```python
from build123d import *

# Parameters (mm, degrees)
ESBO_O1_R                = 2.5
RESSALTO_EXTRUS_O1_DEPTH = 6
ESBO_O2_W                = 13.5
ESBO_O2_H                = 13.5
RESSALTO_EXTRUS_O2_DEPTH = 6
FILETE1_R                = 8
ESBO_O3_R                = 1.5
CORTE_EXTRUS_O1_DEPTH    = 6


with BuildPart() as part:
    # Esboço1 → Ressalto-extrusão1 (new body)
    with BuildSketch(Plane.XY):
        with BuildLine():
            Line((-20, 33.5), (20, 33.5))
            ThreePointArc((20, 33.5), (29.545941546, 29.545941546), (33.5, 20))
            Line((33.5, 20), (33.5, -20))
            ThreePointArc((33.5, -20), (29.545941546, -29.545941546), (20, -33.5))
            Line((20, -33.5), (-20, -33.5))
            ThreePointArc((-20, -33.5), (-29.545941546, -29.545941546), (-33.5, -20))
            Line((-33.5, -20), (-33.5, 20))
            ThreePointArc((-33.5, 20), (-29.545941546, 29.545941546), (-20, 33.5))
        make_face()
        with Locations((-20, 20)):
            Circle(ESBO_O1_R, mode=Mode.SUBTRACT)
        with Locations((20, 20)):
            Circle(ESBO_O1_R, mode=Mode.SUBTRACT)
        with Locations((0, -20)):
            Circle(ESBO_O1_R, mode=Mode.SUBTRACT)
    extrude(amount=RESSALTO_EXTRUS_O1_DEPTH)

    # Esboço2 → Ressalto-extrusão2 (add)
    with BuildSketch(Plane(origin=(0, 0, 0), x_dir=(-1, 0, 0), z_dir=(0, 0, -1))):
        with Locations((-26.75, -26.75)):
            Rectangle(ESBO_O2_W, ESBO_O2_H)
        with Locations((26.75, -26.75)):
            Rectangle(ESBO_O2_W, ESBO_O2_H)
    extrude(amount=-RESSALTO_EXTRUS_O2_DEPTH)

    # Filete1
    filete1_edges = [part.edges().sort_by_distance(p)[0] for p in [
        (33.5, -33.5, 3),
        (-33.5, -33.5, 3),
    ]]
    fillet(filete1_edges, radius=FILETE1_R)

    # Esboço3 → Corte-extrusão1 (cut)
    with BuildSketch(Plane(origin=(0, 0, 0), x_dir=(-1, 0, 0), z_dir=(0, 0, -1))):
        with Locations((0, 20)):
            Circle(ESBO_O3_R)
        with Locations((20, -20)):
            Circle(ESBO_O3_R)
        with Locations((-20, -20)):
            Circle(ESBO_O3_R)
    extrude(amount=-CORTE_EXTRUS_O1_DEPTH, mode=Mode.SUBTRACT)


solid = part.part
```
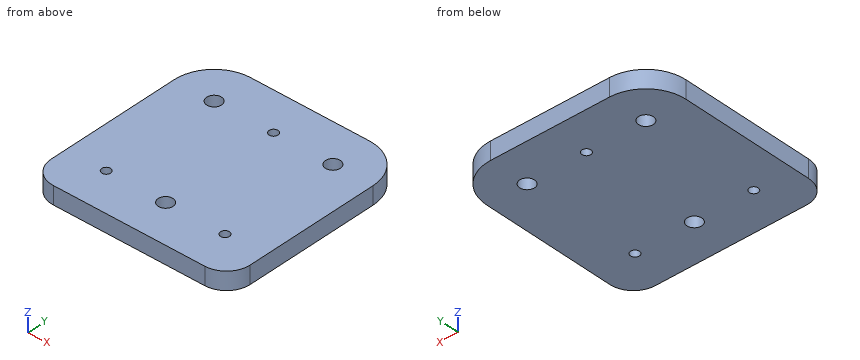
Verification items for the finished model (mm, model axes). Give positions to 0.01 mm unless a question says otherwise; leave off trailing zeros. Order: outer loops, then holes, each group sorted by start corner. A loop starts at its lowest first (then second) coordinate and runs counter-clockwise, first axis right, second up. Notation, with made-up numbers: (67.25, 59.25) -> (111.25, 59.25) arc R18 ccw to (111.25, 64.25) -> close; hole circle Ø3 at (54, 43). An arc over 180 degrees is marked (long way). One line per item, written item: value.
(1) Gauge pin test, flat end, axial feed: pin 1 (1.8 mm diameter, centred on x = 0, y = 20, fed in from -Z). Record the tip position at first contact, or that the pin passes through.
Final values:
pin 1: through
(2) Scan lines: line 1 along Y through (x, z) = (0, 2.85); line 2 along Y through (x, z) = (-20, 4.5); line 3 along X through (y, z) = (-18, 2). Record each from-to range of solid material in increasing order. Write a range as [from, to].
Final values:
line 1: [-33.5, -22.5], [-17.5, 18.5], [21.5, 33.5]
line 2: [-33.5, -21.5], [-18.5, 17.5], [22.5, 33.5]
line 3: [-33.5, -1.5], [1.5, 33.5]
(3) Sectioned sample at B-B on y = -20. Record the cut outline in (x, z).
Final values:
outline: (-33.5, 0) -> (-21.5, 0) -> (-21.5, 6) -> (-33.5, 6) -> close; (-18.5, 0) -> (-2.5, 0) -> (-2.5, 6) -> (-18.5, 6) -> close; (2.5, 0) -> (18.5, 0) -> (18.5, 6) -> (2.5, 6) -> close; (21.5, 0) -> (33.5, 0) -> (33.5, 6) -> (21.5, 6) -> close
(4) Sectioned sample at C-C on z = 2.2. Record the cut outline in (x, y), then the cut area to 3 significant figures.
Final values:
outline: (-33.5, -25.5) arc R8 ccw to (-25.5, -33.5) -> (25.5, -33.5) arc R8 ccw to (33.5, -25.5) -> (33.5, 20) arc R13.5 ccw to (20, 33.5) -> (-20, 33.5) arc R13.5 ccw to (-33.5, 20) -> close; hole circle Ø5 at (-20, 20); hole circle Ø3 at (-20, -20); hole circle Ø5 at (0, -20); hole circle Ø3 at (0, 20); hole circle Ø5 at (20, 20); hole circle Ø3 at (20, -20)
area: 4,300 mm^2
(5) Sectioned sample at A-A on x = 0. Record the cut outline in (y, z), then the cut area to 3 significant figures.
Final values:
outline: (-33.5, 0) -> (-22.5, 0) -> (-22.5, 6) -> (-33.5, 6) -> close; (-17.5, 0) -> (18.5, 0) -> (18.5, 6) -> (-17.5, 6) -> close; (21.5, 0) -> (33.5, 0) -> (33.5, 6) -> (21.5, 6) -> close
area: 354 mm^2
